Verification items for the finished model (mm, model axes). A direction names the side the tool comes from. Coordinates: 2 decimals unless noted, no trailing zeros. Loops run counter-clockwise (first coordinate to the right, second up) from the corner with the lowest first, then second, coordinate; pieces in that order, holes last. Notation, with made-up numbers: (78, -33.5) - (84, -33.5) arc R12 ccw to (84, -14.5) - close; hole circle Ø10 at (60, -5). An arc over 180 degrees is marked (long way). One line per item, written item: value. Start each with the question number.
(1) Set-up check for faces 4 (the face through (2.23, -12.07, -0.22)), 5 (the face through (-2.601, 21.199, 6.676)), 6 (the face through (2.228, -1.124, 8.563)): record each of +Z, -Z, +X, -X, +Y, -Y from which the full face is reachable in a straight line by a thin tool's end or side.
(2) Section check A-A (x = 3). Count the separate pieces of the cut face and the enclosed holes in it, plus the area to 3 significant figures.
(3) Draft check along Z on faces 1 (the face through (-25.56, -11.65, -8.94)), 2 (the face through (38.1, -0.1, -22.5)), 3 (the face through (0.533, -5.506, -24.796)). Enter one of: +Z half, -Z half, draft (parallel to the pull), parting line (faces both ways), or undercut.
(4) Thickness scan on probe 1 along Z at (x, y) = (-3, 0) (3 decimals); probe 2 along Y at (x, z) = (-1, 4); probe 3 along Z at (x, y) = (-6, 1). Record the ranges inside material, lowest first. Write a range as [from, to].
(5) Section check B-B (x = -31.5). Record the boundary of the cut face in (y, z), plus the area to 3 significant figures.
(6) Gauge pin test, flat ends, axial feed: P1, Ø23.5, axis at y = 0, z = 0, coming from the +X side; P2, Ø6, axis at y = 0, z = -17.145, coming from the +X side; P3, Ø9, axis at y = -17.145, z = 0, coming from the +X side. Record the tip position at first contact, or that the pin passes through.
```python
from build123d import *

# Parameters (mm, degrees)
F0_R     = 25.4
F1_DEPTH = 38.1
F2_R     = 22.225
F3_DEPTH = 33.7058
F4_R     = 5.08
F4_R_2   = 8.636
F5_DEPTH = 9.525


with BuildPart() as f1:
    # F0 (on Right) → F1 (new body, symmetric)
    with BuildSketch(Plane.YZ):
        Circle(F0_R)
    extrude(amount=F1_DEPTH, both=True)

    # F2 (on face) → F3 (cut)
    with BuildSketch(Plane.YZ.offset(38.1)):
        Circle(F2_R)
    extrude(amount=-F3_DEPTH, mode=Mode.SUBTRACT)

    # F4 (on face) → F5 (cut)
    with BuildSketch(Plane.YZ.offset(4.3942)):
        with BuildLine():
            ThreePointArc((-7.043346, 12.123346), (-10.179314, 16.816654), (-15.715448, 15.715448))
            ThreePointArc((-15.715448, 15.715448), (-14.067378, 7.430038), (-7.043346, 12.123346))
        make_face()
        with BuildLine():
            ThreePointArc((-12.065, 0), (-17.145, 5.08), (-22.225, 0))
            ThreePointArc((-22.225, 0), (-17.145, -5.08), (-12.065, 0))
        make_face()
        with BuildLine():
            ThreePointArc((-7.043346, -12.123346), (-14.067378, -7.430038), (-15.715448, -15.715448))
            ThreePointArc((-15.715448, -15.715448), (-10.179314, -16.816654), (-7.043346, -12.123346))
        make_face()
        with BuildLine():
            ThreePointArc((5.08, -17.145), (-3.592102, -13.552898), (0, -22.225))
            ThreePointArc((0, -22.225), (3.592102, -20.737102), (5.08, -17.145))
        make_face()
        with BuildLine():
            ThreePointArc((17.203346, -12.123346), (7.430038, -10.179314), (15.715448, -15.715448))
            ThreePointArc((15.715448, -15.715448), (16.816654, -14.067378), (17.203346, -12.123346))
        make_face()
        with Locations((17.145, 0)):
            Circle(F4_R)
        with BuildLine():
            ThreePointArc((17.203346, 12.123346), (16.816654, 14.067378), (15.715448, 15.715448))
            ThreePointArc((15.715448, 15.715448), (7.430038, 10.179314), (17.203346, 12.123346))
        make_face()
        with BuildLine():
            ThreePointArc((0, 22.225), (-3.592102, 13.552898), (5.08, 17.145))
            ThreePointArc((5.08, 17.145), (3.592102, 20.737102), (0, 22.225))
        make_face()
        Circle(F4_R_2)
    extrude(amount=-F5_DEPTH, mode=Mode.SUBTRACT)

    # F6 (on Top) → F7 (revolve, cut)
    with BuildSketch(Plane.XY):
        Polygon((0, 22.225), (-5.1308, 22.225), (-12.671425, 14.684375), (-38.1, 14.684375), (-38.1, 0), (0, 0), align=None)
    revolve(axis=Axis((0, 0, 0), (1, 0, 0)), mode=Mode.SUBTRACT)


solid = f1.part
```
Responses:
1. face 4: +X
1. face 5: none
1. face 6: +X, -X
2. separate pieces: 1
2. enclosed holes: 9
2. area: 1,140 mm²
3. face 1: undercut
3. face 2: draft
3. face 3: parting line
4. probe 1: z = [-25.4, -22.225], [22.225, 25.4]
4. probe 2: y = [-25.08, -21.86], [21.86, 25.08]
4. probe 3: z = [-25.38, -21.33], [21.33, 25.38]
5. outline: circle Ø50.8 at (0, 0); hole circle Ø29.37 at (0, 0)
5. area: 1,350 mm²
6. P1: stops at x = 4.39
6. P2: stops at x = -7.21
6. P3: stops at x = -5.71
